from build123d import *

# Parameters (mm, degrees)
SKETCH1_W           = 43.13
SKETCH1_H           = 17.43
BOSS_EXTRUDE1_DEPTH = 2.7
SKETCH2_W           = 6.47
SKETCH2_H           = 17.43
BOSS_EXTRUDE2_DEPTH = 10.28
SKETCH3_W           = 7.65
SKETCH3_H           = 17.43
BOSS_EXTRUDE3_DEPTH = 10.2
SKETCH4_W           = 18.74
SKETCH4_H           = 17.43
BOSS_EXTRUDE4_DEPTH = 15.4
SKETCH5_W           = 7.411125452
SKETCH5_H           = 17.43
BOSS_EXTRUDE5_DEPTH = 2.54
SKETCH6_W           = 8.4
SKETCH6_H           = 10.28
CUT_EXTRUDE1_DEPTH  = 2.3


with BuildPart() as part:
    # Sketch1 → Boss-Extrude1 (new body)
    with BuildSketch(Plane(origin=(0, 0, 0), x_dir=(1, 0, 0), z_dir=(0, 1, 0))):
        Rectangle(SKETCH1_W, SKETCH1_H)
    extrude(amount=-BOSS_EXTRUDE1_DEPTH)

    # Sketch2 → Boss-Extrude2 (add)
    with BuildSketch(Plane(origin=(0, 0, 0), x_dir=(1, 0, 0), z_dir=(0, 1, 0))):
        with Locations((-18.33, 0)):
            Rectangle(SKETCH2_W, SKETCH2_H)
    extrude(amount=BOSS_EXTRUDE2_DEPTH)

    # Sketch3 → Boss-Extrude3 (add)
    with BuildSketch(Plane(origin=(0, 0, 0), x_dir=(1, 0, 0), z_dir=(0, 1, 0))):
        with Locations((15.975212475, 0)):
            Rectangle(SKETCH3_W, SKETCH3_H)
    extrude(amount=BOSS_EXTRUDE3_DEPTH)

    # Sketch4 → Boss-Extrude4 (add)
    with BuildSketch(Plane(origin=(0, 0, 0), x_dir=(1, 0, 0), z_dir=(0, 1, 0))):
        with Locations((2.780212475, 0)):
            Rectangle(SKETCH4_W, SKETCH4_H)
    extrude(amount=BOSS_EXTRUDE4_DEPTH)

    # Sketch5 → Boss-Extrude5 (add)
    with BuildSketch(Plane(origin=(0, 0, 0), x_dir=(1, 0, 0), z_dir=(0, 1, 0))):
        with Locations((-10.86460908, 0)):
            Rectangle(SKETCH5_W, SKETCH5_H)
    extrude(amount=BOSS_EXTRUDE5_DEPTH)

    # Sketch6 → Cut-Extrude1 (cut)
    with BuildSketch(Plane.ZY.offset(21.565)):
        with Locations((0, 5.14)):
            Rectangle(SKETCH6_W, SKETCH6_H)
    extrude(amount=-CUT_EXTRUDE1_DEPTH, mode=Mode.SUBTRACT)


solid = part.part
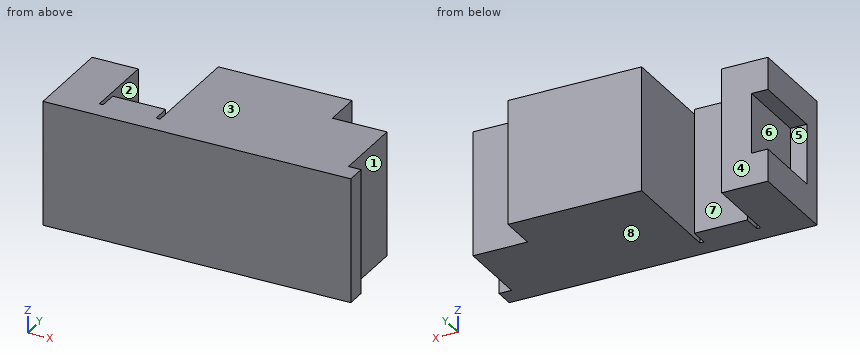
Verification items for the finished model (mm, model axes). Face numbers are marked on the shaded views. A direction names the side the tool comes from. Give positions to 0.01 mm unless a question says otherwise; leave off trailing zeros. Order: outer loops, then holes, each group sorted by start corner. A loop starts at its lowest first (then second) coordinate and runs counter-clockwise, first axis right, second up. Notation, with made-up numbers: M -35,89.5 L -8,89.5 A23 ccw -8,111.5 Z; hole C -4.5,33.25 d9. An arc over 180 degrees is marked long. Answer as a JSON object with one key per item and string values. Group by question number.
1) Access from +Z, -Z, +X, -X, +Y, -Y to the whole of each face (thin tool, end or side, straight path). Record for the marked faces 1, 2, 3, 4 and 5.
2) Cross-section at B-B (y = 1.25). Enter the section's corners in (x, z) (3 decimals), then the cut area to 3 significant figures.
3) Depth check by flat-ended pin: pin 1 Ø8.5 at (x, z) = (17, -0.5) entering from +Y; pin 2 Ø1.9 at (x, z) = (-17, -0.5) entering from +Y; pin 3 Ø1.2 at (x, z) = (-20.5, -0.5) entering from +Y. Enter the tip coordinate at first touch or a pass-through.
4) Mould release check, pull along Z, two halves, no side actions. Record for the marked faces 6, 7 and 8: released by +Z, released by -Z, zero draft, split by the parting line, or undercut.
5) Cross-section at C-C (z = -6). Enter the section's corners in (x, y) (3 decimals), then the cut area to 3 significant figures.
6) Cross-section at D-D (x = -18). Enter the section's corners in (y, z) (3 decimals).
7) Cross-section at A-A (y = 6.25). Enter the section's corners in (x, z) (3 decimals), then the cut area to 3 significant figures.
8) Scan lines: line 1 along X through (y, z) = (0.75, 6.5) (3 decimals); line 2 along X through (y, z) = (4.5, -1) (3 decimals); line 3 along X through (y, z) = (7.5, -4.25) (3 decimals). Record each from-to range of solid material in increasing order. Write a range as [from, to].
Result sheet:
{
 "1": {"face 1": "+Z, -Z, +X, +Y", "face 2": "+Z, -Z, +Y", "face 3": "+Z, +X, -X, +Y, -Y", "face 4": "+Z, -Z, -X, +Y", "face 5": "-X, +Y"},
 "2": {"outline": "M -21.565,-8.715 L -15.095,-8.715 L -15.095,8.715 L -21.565,8.715 L -21.565,4.2 L -19.265,4.2 L -19.265,-4.2 L -21.565,-4.2 Z; M -14.57,-8.715 L -7.159,-8.715 L -7.159,8.715 L -14.57,8.715 Z; M -6.59,-8.715 L 19.8,-8.715 L 19.8,8.715 L -6.59,8.715 Z", "area": "683 mm2"},
 "3": {"pin 1": "stops at y = 10.2", "pin 2": "stops at y = 10.28", "pin 3": "stops at y = 0"},
 "4": {"face 6": "undercut", "face 7": "zero draft", "face 8": "released by -Z"},
 "5": {"outline": "M -21.565,-2.7 L 21.565,-2.7 L 21.565,0 L 19.8,0 L 19.8,10.2 L 12.15,10.2 L 12.15,15.4 L -6.59,15.4 L -6.59,0 L -7.159,0 L -7.159,2.54 L -14.57,2.54 L -14.57,0 L -15.095,0 L -15.095,10.28 L -21.565,10.28 Z", "area": "568 mm2"},
 "6": {"outline": "M -2.7,-8.715 L 10.28,-8.715 L 10.28,8.715 L -2.7,8.715 Z"},
 "7": {"outline": "M -21.565,-8.715 L -15.095,-8.715 L -15.095,8.715 L -21.565,8.715 L -21.565,4.2 L -19.265,4.2 L -19.265,-4.2 L -21.565,-4.2 Z; M -6.59,-8.715 L 19.8,-8.715 L 19.8,8.715 L -6.59,8.715 Z", "area": "553 mm2"},
 "8": {"line 1": "x = [-21.565, -15.095], [-14.57, -7.159], [-6.59, 19.8]", "line 2": "x = [-19.265, -15.095], [-6.59, 19.8]", "line 3": "x = [-21.565, -15.095], [-6.59, 19.8]"}
}
